Design review of the part built by this model. Coordinates are the model's own, in mm. A direction names the side the tool comes from. Give positions to 0.01 mm unless a question says otherwise; leave off trailing zeros. Write each loop counter-clockwise with the first axis right and the second up, starting at its lowest first coordinate (ties: lowest second). Pieces come first, ordered by that corner, then holes. Notation, with made-up numbers: M 41,56.5 L 85,56.5 A21 cw 85,87.5 Z; hole C -31.5,88.5 d6. An arc over 180 degrees is marked long. Use one line per item in the form item = value. Start each with the question number.
Autodesk Fusion 360 part; units mm, degrees
sketch "Skizze1" plane through (0, 0, 0) normal (0, 0, 1) x (1, 0, 0)
  line L0 (0, 0) -> (107, 0)
  line L1 (107, 0) -> (107, 135.5)
  line L2 (107, 135.5) -> (0, 135.5)
  line L3 (0, 135.5) -> (0, 0)
  dimension "d1" = 107
  dimension "d2" = 135.5
extrude "Extrusion1" add sketch "Skizze1" along normal blind 3
sketch "Skizze2" plane through (0, 0, 3) normal (0, 0, 1) x (-1, 0, 0)
  line L0 (0, -135.5) -> (0, 0)
  line L1 (0, 0) -> (-107, 0)
  line L2 (-107, 0) -> (-107, -135.5)
  line L3 (-107, -135.5) -> (0, -135.5)
  line L4 (-22, -41) -> (-85, -41)
  line L5 (-85, -41) -> (-85, -94.5)
  line L6 (-85, -94.5) -> (-22, -94.5)
  line L7 (-22, -94.5) -> (-22, -41)
  circle A0 centre (-53.5, -41) radius 17.5
  circle A1 centre (-53.5, -94.5) radius 17.5
  dimension "d5" = 63
  dimension "d6" = 53.5
  dimension "d7" = 41
  dimension "d8" = 22
  dimension "d9" = 35
  dimension "d10" = 35
extrude "Extrusion2" cut sketch "Skizze2" against normal blind 2 contours L4 L5 L6 L7 A0 A1 | L4 A0 | L4 A0 | L6 A1 | L6 A1
sketch "Skizze3" plane through (0, 0, 0) normal (0, 0, -1) x (1, 0, 0)
  line L0 (0, 0) -> (0, -135.5)
  line L1 (0, -135.5) -> (107, -135.5)
  line L2 (107, -135.5) -> (107, 0)
  line L3 (107, 0) -> (0, 0)
  line L4 (0, 0) -> (7, 0)
  line L5 (7, 0) -> (7, -7)
  line L6 (7, -7) -> (0, -7)
  line L7 (0, -7) -> (0, 0)
  line L8 (107, 0) -> (100, 0)
  line L9 (100, 0) -> (100, -7)
  line L10 (100, -7) -> (107, -7)
  line L11 (107, -7) -> (107, 0)
  line L12 (0, -135.5) -> (7, -135.5)
  line L13 (7, -135.5) -> (7, -128.5)
  line L14 (7, -128.5) -> (0, -128.5)
  line L15 (0, -128.5) -> (0, -135.5)
  line L16 (107, -135.5) -> (100, -135.5)
  line L17 (100, -135.5) -> (100, -128.5)
  line L18 (100, -128.5) -> (107, -128.5)
  line L19 (107, -128.5) -> (107, -135.5)
  circle A0 centre (3.5, -132) radius 2.65
  circle A1 centre (103.5, -132) radius 2.65
  circle A2 centre (103.5, -3.5) radius 2.65
  circle A3 centre (3.5, -3.5) radius 2.65
  dimension "d13" = 7
  dimension "d14" = 7
  dimension "d15" = 7
  dimension "d16" = 7
  dimension "d17" = 7
  dimension "d18" = 7
  dimension "d19" = 7
  dimension "d20" = 7
  dimension "d21" = 5.3
  dimension "d22" = 5.3
  dimension "d23" = 5.3
  dimension "d24" = 5.3
  dimension "d25" = 3.5
  dimension "d26" = 3.5
  dimension "d27" = 3.5
  dimension "d28" = 3.5
  dimension "d29" = 3.5
  dimension "d30" = 3.5
  dimension "d31" = 3.5
  dimension "d32" = 3.5
extrude "Extrusion3" cut sketch "Skizze3" against normal blind 1.2 contours A0 | A1 | A2 | A3
fillet "Abrundung1" radius 2 4 edges at (107, 0, 1.5) (107, 135.5, 1.5) (0, 135.5, 1.5) (0, 0, 1.5)
equation "d7 = 44 mm - 3 mm"
1. We need section D-D (x = 3.5). State the section outline as (y, z) points.
2. Clearance check with flat-ended pins moving along their axes: pin 1 Ø4 at (x, y) = (36.5, 78) entering from +Z; pin 2 Ø1.6 at (x, y) = (2, 4) entering from -Z. State where each tip first meets the part, or that it passes through.
3. We need section A-A (z = 1.85). State the section outline as (x, y) points.
4. We need section B-B (y = 55.5). State the section outline as (x, z) points.
5. Draft analysis for pull direction X (two halves, no side actions). For faces 4 (the flat face through (0, 69, 1)), 5 (the cylindrical face through (53.885, 111.996, 2.014)), 6 (the flat face through (17, 69, 3)), state which applies: pulls with the +X half, pulls with the -X half, needs draft (parallel to the pull), parting line crosses it, or undercut.
6. To check wall thickness, follow L1, parallel to X at y = 132, z = 0.9; L2, parallel to Y at x = 3.5, z = 0.9; L3, parallel to X at y = 44, z = 1.4. State the ranges of each line that lie inside material, in increasing order.
7. We need section C-C (x = 27). State the section outline as (y, z) points.
8. For faces 1 (the flat face through (103, 132, 1.2)), 2 (the flat face through (54, 67, 1)), 3 (the flat face through (53, 0, 1)), list the 3-axis set-ups (+Z, -Z, +X, -X, +Y, -Y) from which the entire face can be reached by the end or side of a thin tool; tool diameter is ignored.
Answer block:
q1.outline = M 0,0 L 0.85,0 L 0.85,1.2 L 6.15,1.2 L 6.15,0 L 129.35,0 L 129.35,1.2 L 134.65,1.2 L 134.65,0 L 135.5,0 L 135.5,3 L 0,3 Z
q2.pin_1 = 1
q2.pin_2 = 1.2
q3.outline = M 0,2 A2 ccw 2,0 L 105,0 A2 ccw 107,2 L 107,133.5 A2 ccw 105,135.5 L 2,135.5 A2 ccw 0,133.5 Z; hole M 22,41 L 36,41 A17.5 ccw 71,41 L 85,41 L 85,94.5 L 71,94.5 A17.5 ccw 36,94.5 L 22,94.5 Z
q4.outline = M 0,0 L 107,0 L 107,3 L 85,3 L 85,1 L 22,1 L 22,3 L 0,3 Z
q5.face_4 = pulls with the -X half
q5.face_5 = undercut
q5.face_6 = needs draft
q6.L1 = 0 to 0.85, 6.15 to 100.85, 106.15 to 107
q6.L2 = 0 to 0.85, 6.15 to 129.35, 134.65 to 135.5
q6.L3 = 0 to 22, 85 to 107
q7.outline = M 0,0 L 135.5,0 L 135.5,3 L 94.5,3 L 94.5,1 L 41,1 L 41,3 L 0,3 Z
q8.face_1 = -Z
q8.face_2 = +Z
q8.face_3 = +Z, -Z, +X, -X, -Y
